from build123d import *

# Parameters (mm, degrees)
EXTRUDE_5_DEPTH     = 118
SKETCH_8_R          = 45
CUT_EXTRUDE_2_DEPTH = 130
CHAMFER_1_SIZE      = 6
SKETCH_9_W          = 30
SKETCH_9_H          = 78
CUT_EXTRUDE_3_DEPTH = 130
CHAMFER_2_SIZE      = 5
CHAMFER_3_SIZE      = 5
SKETCH_10_R         = 2.75
CUT_EXTRUDE_4_DEPTH = 146.163700697
SKETCH_14_R         = 1.9
CUT_EXTRUDE_5_DEPTH = 146.163700697
SKETCH_15_R         = 3.5
CUT_EXTRUDE_6_DEPTH = 2


with BuildPart() as part:
    # 草图7 → 凸台-拉伸5 (new body)
    with BuildSketch(Plane(origin=(0, 0, 0), x_dir=(1, 0, 0), z_dir=(0, 1, 0))):
        Polygon((-67.5, 0), (67.5, 0), (67.5, -18.5), (82.5, -18.5), (82.5, -23.5), (60, -23.5), (60, -5), (-60, -5), (-60, -23.5), (-82.5, -23.5), (-82.5, -18.5), (-67.5, -18.5), align=None)
    extrude(amount=EXTRUDE_5_DEPTH)

    # 草图8 → 切除-拉伸2 (cut)
    with BuildSketch(Plane(origin=(0, 0, 0), x_dir=(-1, 0, 0), z_dir=(0, 0, -1))):
        with Locations((0, 59)):
            Circle(SKETCH_8_R)
    extrude(amount=-CUT_EXTRUDE_2_DEPTH, mode=Mode.SUBTRACT)

    # 倒角1
    chamfer_1_edges = [part.edges().sort_by_distance(p)[0] for p in [
        (82.5, 0, 21),
        (-82.5, 0, 21),
        (-82.5, 118, 21),
        (82.5, 118, 21),
    ]]
    chamfer(chamfer_1_edges, length=CHAMFER_1_SIZE)

    # 草图9 → 切除-拉伸3 (cut)
    with BuildSketch(Plane(origin=(0, 0, 18.5), x_dir=(-1, 0, 0), z_dir=(0, 0, -1))):
        with Locations((-82.5, 59)):
            Rectangle(SKETCH_9_W, SKETCH_9_H)
        with Locations((82.5, 59)):
            Rectangle(SKETCH_9_W, SKETCH_9_H)
    extrude(amount=-CUT_EXTRUDE_3_DEPTH, mode=Mode.SUBTRACT)

    # 倒角2
    chamfer_2_edges = [part.edges().sort_by_distance(p)[0] for p in [
        (-67.5, 59, 0),
        (67.5, 59, 0),
    ]]
    chamfer(chamfer_2_edges, length=CHAMFER_2_SIZE)

    # 倒角3
    chamfer_3_edges = [part.edges().sort_by_distance(p)[0] for p in [
        (60, 59, 5),
        (-60, 59, 5),
    ]]
    chamfer(chamfer_3_edges, length=CHAMFER_3_SIZE)

    # 草图10 → 切除-拉伸4 (cut, through all)
    with BuildSketch(Plane(origin=(0, 0, 18.5), x_dir=(-1, 0, 0), z_dir=(0, 0, -1))):
        with Locations((75, 10)):
            Circle(SKETCH_10_R)
        with Locations((-75, 10)):
            Circle(SKETCH_10_R)
        with Locations((-75, 108)):
            Circle(SKETCH_10_R)
        with Locations((75, 108)):
            Circle(SKETCH_10_R)
    extrude(amount=-CUT_EXTRUDE_4_DEPTH, mode=Mode.SUBTRACT)

    # 草图14 → 切除-拉伸5 (cut, through all)
    with BuildSketch(Plane.XY.offset(5)):
        with Locations((-37.123106012, 96.123106012)):
            Circle(SKETCH_14_R)
        with Locations((-37.123106012, 21.876893988)):
            Circle(SKETCH_14_R)
        with Locations((37.123106012, 21.876893988)):
            Circle(SKETCH_14_R)
        with Locations((37.123106012, 96.123106012)):
            Circle(SKETCH_14_R)
    extrude(amount=-CUT_EXTRUDE_5_DEPTH, mode=Mode.SUBTRACT)

    # 草图15 → 切除-拉伸6 (cut)
    with BuildSketch(Plane.XY.offset(5)):
        with Locations((-37.123106012, 96.123106012)):
            Circle(SKETCH_15_R)
        with Locations((37.123106012, 96.123106012)):
            Circle(SKETCH_15_R)
        with Locations((37.123106012, 21.876893988)):
            Circle(SKETCH_15_R)
        with Locations((-37.123106012, 21.876893988)):
            Circle(SKETCH_15_R)
    extrude(amount=-CUT_EXTRUDE_6_DEPTH, mode=Mode.SUBTRACT)


solid = part.part
Design review of the part built by this model. Coordinates are the model's own, in mm. A direction names the side the tool comes from. Coordinates: 2 decimals unless noted, no trailing zeros. Loops run counter-clockwise (first coordinate to the right, second up) from the corner with the lowest first, then second, coordinate; pieces in that order, holes last. Notation, with made-up numbers: (2.25, -4.5) - (7.25, -4.5) arc R10 cw to (7.25, 10.5) - close; hole circle Ø3 at (72, 83.25). An arc over 180 degrees is marked (long way). Use CSV: the item, a comma, the result in double quotes. Start each with the question number.
1. Add section A-A on x = -70.5. Give the boundary of the cut face in (y, z).
2. To check wall thickness, follow probe 1 along Y at (x, z) = (-75, 20.75); probe 2 along X at (y, z) = (113, 12.5); probe 3 along X at (y, z) = (102.5, 19.5). State the ranges of each line that lie inside material, in increasing order.
3. For faces 4 (the flat face through (-82.5, 105, 21)), 5 (the flat face through (-76.8, 105.6, 18.5)), 6 (the flat face through (60, 58, 17)), 7 (the flat face through (-35.6, 94.6, 3)), list the 3-axis set-ups (+Z, -Z, +X, -X, +Y, -Y) from which the entire face can be reached by the end or side of a thin tool; tool diameter is ignored.
4. Add section C-C on z = 16.25. Give the boundary of the cut face in (x, y), plus the area to 3 significant figures.
5. Clearance check with flat-ended pins moving along their axes: pin 1 (5 mm diameter, centred on x = 35, y = 91, fed in from -Z); pin 2 (2.5 mm diameter, centred on x = 37.12, y = 96.12, fed in from -Z); pin 3 (4 mm diameter, centred on y = 60, z = 14.5, fed in from -X); pin 4 (12 mm diameter, centred on x = 74.5, y = 105.5, fed in from -Z). State where each tip first meets the part, or that it passes through.
6. Add section D-D on y = 59. Give the boundary of the cut face in (x, z), plus the area to 4 significant figures.
7. Add section B-B on y = 10. Give the boundary of the cut face in (x, z).
8. Mouldability with a two-part tool opening along Y and no side actions: class faces 1 (the flat face through (79.5, 115, 21)), 2 (the cylindrical face through (77.182, 106.327, 20.965)), 3 (the flat face through (82.5, 13, 21)) as released by +Y, released by -Y, zero draft, split by the parting line, or undercut.
Resolved:
1,outline,"(0, 18.5) - (20, 18.5) - (20, 23.5) - (0, 23.5) - close; (98, 18.5) - (118, 18.5) - (118, 23.5) - (98, 23.5) - close"
2,probe 1,"0 to 7.25, 12.75 to 20, 98 to 105.25, 110.75 to 118"
2,probe 2,"-67.5 to -60, 60 to 67.5"
2,probe 3,"-82.5 to -60, 60 to 82.5"
3,face 4,"+Z, -Z, -X, +Y, -Y"
3,face 5,"-Z, -X, +Y, -Y"
3,face 6,"+Z, +Y, -Y"
3,face 7,"+Z"
4,outline,"(-67.5, 0) - (-60, 0) - (-60, 118) - (-67.5, 118) - close; (60, 0) - (67.5, 0) - (67.5, 118) - (60, 118) - close"
4,area,"1,770 mm2"
5,pin 1,"z = 0"
5,pin 2,"through"
5,pin 3,"x = -67.5"
5,pin 4,"z = 18.5"
6,outline,"(-67.5, 5) - (-62.5, 0) - (-45, 0) - (-45, 5) - (-55, 5) - (-60, 10) - (-60, 23.5) - (-67.5, 23.5) - close; (45, 0) - (62.5, 0) - (67.5, 5) - (67.5, 23.5) - (60, 23.5) - (60, 10) - (55, 5) - (45, 5) - close"
6,area,"502.5 mm2"
7,outline,"(-82.5, 18.5) - (-77.75, 18.5) - (-77.75, 23.5) - (-82.5, 23.5) - close; (-72.25, 18.5) - (-67.5, 18.5) - (-67.5, 5) - (-62.5, 0) - (62.5, 0) - (67.5, 5) - (67.5, 18.5) - (72.25, 18.5) - (72.25, 23.5) - (60, 23.5) - (60, 10) - (55, 5) - (-55, 5) - (-60, 10) - (-60, 23.5) - (-72.25, 23.5) - close; (77.75, 18.5) - (82.5, 18.5) - (82.5, 23.5) - (77.75, 23.5) - close"
8,face 1,"released by +Y"
8,face 2,"undercut"
8,face 3,"zero draft"
